CAD build for the part. Positions are in the model's coordinates, mm. A direction names the side the tool comes from. Round coordinates to 2 decimals unless told otherwise and drop trailing zeros. Order: outer loops, then holes, each group sorted by start corner. A loop starts at its lowest first (then second) coordinate and runs counter-clockwise, first axis right, second up. Notation, with made-up numbers: M 33,-7 L 64,-7 A10 cw 64,10 Z; hole C 68,0.25 d5. An arc over 180 degrees is marked long. Answer as a JSON object with one key per item and string values.
```python
from build123d import *

# Parameters (mm, degrees)
F0_W     = 42.2
F0_H     = 12
F0_R     = 2
F0_W_2   = 5
F1_DEPTH = 5
F2_DEPTH = 15
F3_W     = 12
F3_H     = 5
F4_DEPTH = 10
F5_W     = 12
F5_H     = 5
F6_DEPTH = 10
F7_R     = 2
F8_DEPTH = 5
F9_DEPTH = 2


with BuildPart() as f1:
    # F0 (on Top) → F1 (new body)
    with BuildSketch(Plane.XY):
        Rectangle(F0_W, F0_H)
        with Locations((-15.5, 0)):
            Circle(F0_R, mode=Mode.SUBTRACT)
        with Locations((15.5, 0)):
            Circle(F0_R, mode=Mode.SUBTRACT)
        with Locations((23.6, 0)):
            Rectangle(F0_W_2, F0_H)
        with Locations((-23.6, 0)):
            Rectangle(F0_W_2, F0_H)
    extrude(amount=F1_DEPTH)

    # F0 (on Top) → F2 (join)
    with BuildSketch(Plane.XY):
        with Locations((23.6, 0)):
            Rectangle(F0_W_2, F0_H)
        with Locations((-23.6, 0)):
            Rectangle(F0_W_2, F0_H)
    extrude(amount=-F2_DEPTH)

    # F3 (on face) → F4 (join)
    with BuildSketch(Plane(origin=(-26.1, 0, 0), x_dir=(0, -1, 0), z_dir=(-1, 0, 0))):
        with Locations((0, -12.5)):
            Rectangle(F3_W, F3_H)
    extrude(amount=F4_DEPTH)

    # F5 (on face) → F6 (join)
    with BuildSketch(Plane.YZ.offset(26.1)):
        with Locations((0, -12.5)):
            Rectangle(F5_W, F5_H)
    extrude(amount=F6_DEPTH)

    # F7 (on face) → F8 (cut)
    with BuildSketch(Plane.XY.offset(-10)):
        with Locations((31.1, 0)):
            Circle(F7_R)
        with Locations((-31.1, 0)):
            Circle(F7_R)
    extrude(amount=-F8_DEPTH, mode=Mode.SUBTRACT)

    # F7 (on face) → F9 (cut)
    with BuildSketch(Plane.XY.offset(-10)):
        Polygon((28.1, 1.732051), (28.1, -1.732051), (31.1, -3.464102), (34.1, -1.732051), (34.1, 1.732051), (31.1, 3.464102), align=None)
        with Locations((31.1, 0)):
            Circle(F7_R, mode=Mode.SUBTRACT)
        Polygon((-34.1, -1.732051), (-31.1, -3.464102), (-28.1, -1.732051), (-28.1, 1.732051), (-31.1, 3.464102), (-34.1, 1.732051), align=None)
        with Locations((-31.1, 0)):
            Circle(F7_R, mode=Mode.SUBTRACT)
    extrude(amount=-F9_DEPTH, mode=Mode.SUBTRACT)


solid = f1.part
```
Item 1: 3-axis set-ups, long thin cutter, end or side, ignore diameter. For faces 4 (the cylindrical face through (-33.098, 0.088, -13.479)), 5 (the flat face through (-21.1, 0, -7)), 6 (the flat face through (29.6, -2.6, -11)), 7 (the flat face through (26.1, 0, -2)): which of +Z, -Z, +X, -X, +Y, -Y reach the whole face in a straight line?
Worked answers:
{"face 4": "+Z, -Z", "face 5": "-Z, +Y, -Y", "face 6": "+Z", "face 7": "+Z, +X, +Y, -Y"}
Item 2: Wall check: line 1 along Y through (x, z) = (31.1, -12.8); line 2 along X through (y, z) = (-2, -3.75); line 3 along X through (y, z) = (1.5, 4.25). Give the ranges that are in metal, low to high. Write a range as [from, to].
Worked answers:
{"line 1": "y = [-6, -2], [2, 6]", "line 2": "x = [-26.1, -21.1], [21.1, 26.1]", "line 3": "x = [-26.1, -16.82], [-14.18, 14.18], [16.82, 26.1]"}
Item 3: Drop flat-ended pins along their axis: pin 1 Ø3 at (x, y) = (15.5, 0) entering from -Z; pin 2 Ø4 at (y, z) = (1.5, -0.5) entering from +X; pin 3 Ø6.5 at (x, y) = (-32.5, -1) entering from +Z; pin 4 Ø3.5 at (y, z) = (-2, -4) entering from -X. Give the stop position or say it passes through.
Worked answers:
{"pin 1": "passes through", "pin 2": "stops at x = 26.1", "pin 3": "stops at z = -10", "pin 4": "stops at x = -26.1"}
Item 4: Saw through at D-D on x = 0. List the corners of the cut face in (y, z), and give its area (3 significant figures).
Worked answers:
{"outline": "M -6,0 L 6,0 L 6,5 L -6,5 Z", "area": "60.0 mm2"}
Item 5: Saw through at B-B on x = -15.5. List the corners of the cut face in (y, z).
Worked answers:
{"outline": "M -6,0 L -2,0 L -2,5 L -6,5 Z; M 2,0 L 6,0 L 6,5 L 2,5 Z"}
Item 6: Saw through at C-C on z = -8.5. List the corners of the cut face in (x, y), and give its area (3 significant figures).
Worked answers:
{"outline": "M -26.1,-6 L -21.1,-6 L -21.1,6 L -26.1,6 Z; M 21.1,-6 L 26.1,-6 L 26.1,6 L 21.1,6 Z", "area": "120 mm2"}
Item 7: Two-plate mould, pull along Y, no slides. Class faces 1 (the flat face through (-1, -6, 2)), 2 (the flat face through (-26.1, 0, -3)), 3 (the flat face through (34.1, 0, -11)): released by +Y, released by -Y, zero draft, split by the parting line, or undercut.
Worked answers:
{"face 1": "released by -Y", "face 2": "zero draft", "face 3": "undercut"}
Item 8: Saw through at A-A on z = -13.25. List the corners of the cut face in (x, y), and give its area (3 significant figures).
Worked answers:
{"outline": "M -36.1,-6 L -21.1,-6 L -21.1,6 L -36.1,6 Z; M 21.1,-6 L 36.1,-6 L 36.1,6 L 21.1,6 Z; hole C -31.1,0 d4; hole C 31.1,0 d4", "area": "335 mm2"}
